Job drawing, mm, ordinate dimensions from the low corner. One solid piece. Coordinates: 2 decimals unless noted, no trailing zeros. Order: outer loops, then holes, each group sorted by start corner. A loop starts at its lowest first (then second) coordinate and runs counter-clockwise, first axis right, second up. Notation, with made-up numbers: M -16.5,18.25 L 39.5,18.25 A20 ccw 39.5,43.25 Z; hole C 76.5,42 d10. An arc over 180 degrees is marked long. Write item = value, one per line. Start each with the question number.
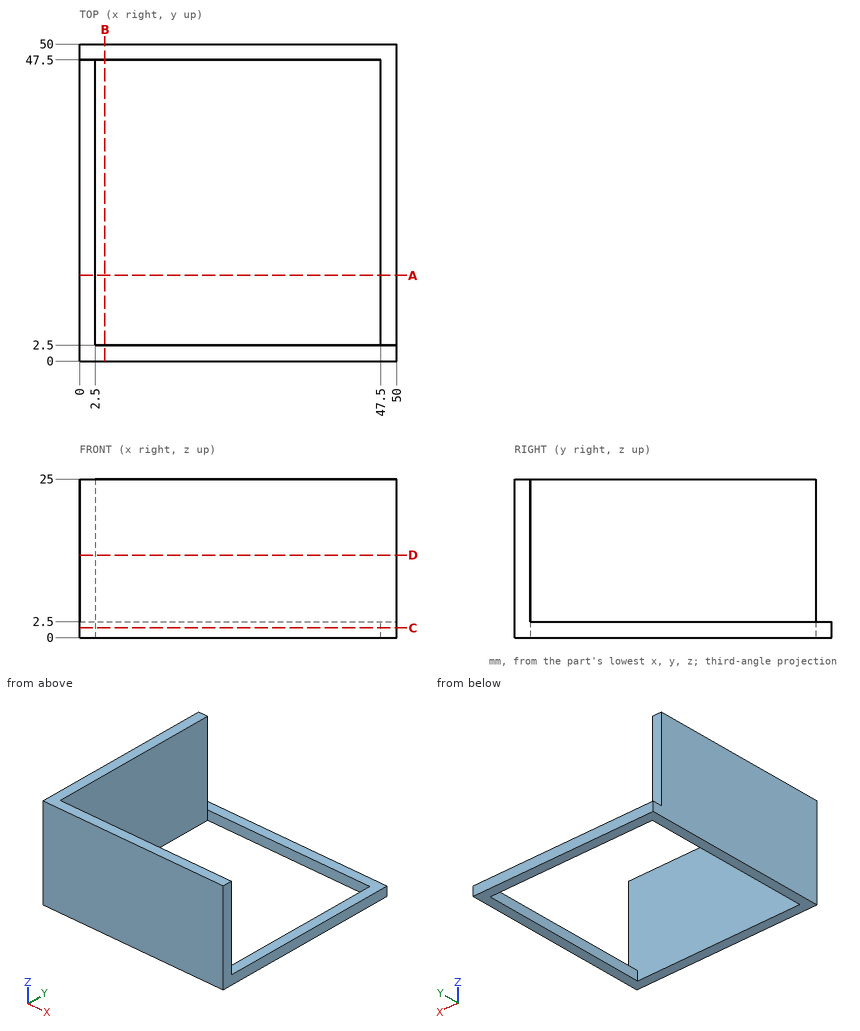
1. Slice it at A-A (y = 13.5). Write the cut outline in (x, z).
2. Slice it at C-C (z = 1.5). Write the cut outline in (x, y).
3. Slice it at D-D (z = 13). Write the cut outline in (x, y), plus the area to 4 significant figures.
4. Probe L1, parallel to X at y = 6, z = 1.25; L2, parallel to X at y = 45, z = 4.75. List the from-to ranges inside material, lowest first.
5. Flat gauge pins, fed straight in: pin 1 (10 mm diameter, centred on y = 16.5, z = 8.5, fed in from +X); pin 2 (0.8 mm diameter, centred on x = 1, z = 11, fed in from +Y); pin 3 (1.5 mm diameter, centred on x = 13, z = 16.5, fed in from +Y). Where does each tip first touch, or does it go through?
Calculated:
q1.outline = M 0,0 L 2.5,0 L 2.5,25 L 0,25 Z; M 47.5,0 L 50,0 L 50,2.5 L 47.5,2.5 Z
q2.outline = M 0,0 L 50,0 L 50,50 L 0,50 Z; hole M 2.5,2.5 L 47.5,2.5 L 47.5,47.5 L 2.5,47.5 Z
q3.outline = M 0,0 L 50,0 L 50,2.5 L 2.5,2.5 L 2.5,47.5 L 0,47.5 Z
q3.area = 237.5 mm²
q4.L1 = 0 to 2.5, 47.5 to 50
q4.L2 = 0 to 2.5
q5.pin_1 = 2.5
q5.pin_2 = 47.5
q5.pin_3 = 2.5
